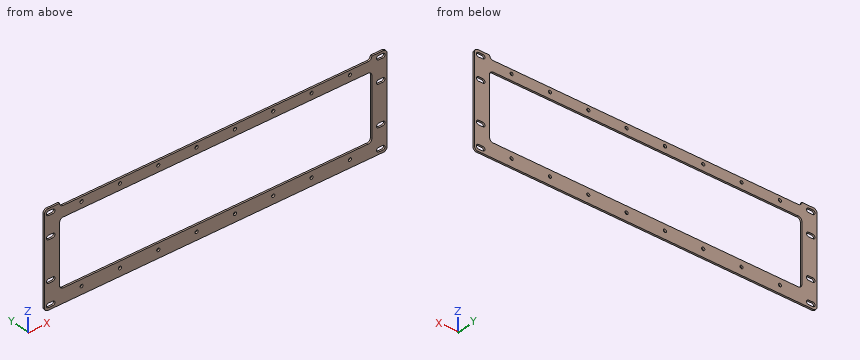
from build123d import *

# Parameters (mm, degrees)
F1_R     = 2.25
F2_DEPTH = 2.5


with BuildPart() as f2:
    # F1 (on face) → F2 (new body)
    with BuildSketch(Plane.XZ):
        with BuildLine():
            Line((241.3, -61.675), (241.3, 61.675))
            ThreePointArc((241.3, 61.675), (239.8355339059, 65.2105339059), (236.3, 66.675))
            Line((236.3, 66.675), (220, 66.675))
            ThreePointArc((220, 66.675), (218.5355339059, 63.1394660941), (215, 61.675))
            Line((215, 61.675), (-215, 61.675))
            ThreePointArc((-215, 61.675), (-218.5355339059, 63.1394660941), (-220, 66.675))
            Line((-220, 66.675), (-236.3, 66.675))
            ThreePointArc((-236.3, 66.675), (-239.8355339059, 65.2105339059), (-241.3, 61.675))
            Line((-241.3, 61.675), (-241.3, -61.675))
            ThreePointArc((-241.3, -61.675), (-239.8355339059, -65.2105339059), (-236.3, -66.675))
            Line((-236.3, -66.675), (236.3, -66.675))
            ThreePointArc((236.3, -66.675), (239.8355339059, -65.2105339059), (241.3, -61.675))
        make_face()
        with BuildLine():
            Line((-235.5, -57.4), (-229.5, -57.4))
            ThreePointArc((-229.5, -57.4), (-226.5, -60.4), (-229.5, -63.4))
            Line((-229.5, -63.4), (-235.5, -63.4))
            ThreePointArc((-235.5, -63.4), (-238.5, -60.4), (-235.5, -57.4))
        make_face(mode=Mode.SUBTRACT)
        with Locations((-189, -55.5)):
            Circle(F1_R, mode=Mode.SUBTRACT)
        with Locations((-135, -55.5)):
            Circle(F1_R, mode=Mode.SUBTRACT)
        with Locations((-81, -55.5)):
            Circle(F1_R, mode=Mode.SUBTRACT)
        with Locations((-27, -55.5)):
            Circle(F1_R, mode=Mode.SUBTRACT)
        with BuildLine():
            Line((-235.5, -25.6), (-229.5, -25.6))
            ThreePointArc((-229.5, -25.6), (-226.5, -28.6), (-229.5, -31.6))
            Line((-229.5, -31.6), (-235.5, -31.6))
            ThreePointArc((-235.5, -31.6), (-238.5, -28.6), (-235.5, -25.6))
        make_face(mode=Mode.SUBTRACT)
        with Locations((27, -55.5)):
            Circle(F1_R, mode=Mode.SUBTRACT)
        with Locations((81, -55.5)):
            Circle(F1_R, mode=Mode.SUBTRACT)
        with Locations((135, -55.5)):
            Circle(F1_R, mode=Mode.SUBTRACT)
        with BuildLine():
            Line((229.5, -57.4), (235.5, -57.4))
            ThreePointArc((235.5, -57.4), (238.5, -60.4), (235.5, -63.4))
            Line((235.5, -63.4), (229.5, -63.4))
            ThreePointArc((229.5, -63.4), (226.5, -60.4), (229.5, -57.4))
        make_face(mode=Mode.SUBTRACT)
        with Locations((189, -55.5)):
            Circle(F1_R, mode=Mode.SUBTRACT)
        with BuildLine():
            Line((229.5, -25.6), (235.5, -25.6))
            ThreePointArc((235.5, -25.6), (238.5, -28.6), (235.5, -31.6))
            Line((235.5, -31.6), (229.5, -31.6))
            ThreePointArc((229.5, -31.6), (226.5, -28.6), (229.5, -25.6))
        make_face(mode=Mode.SUBTRACT)
        with BuildLine():
            Line((-235.5, 31.6), (-229.5, 31.6))
            ThreePointArc((-229.5, 31.6), (-226.5, 28.6), (-229.5, 25.6))
            Line((-229.5, 25.6), (-235.5, 25.6))
            ThreePointArc((-235.5, 25.6), (-238.5, 28.6), (-235.5, 31.6))
        make_face(mode=Mode.SUBTRACT)
        with Locations((-189, 55.5)):
            Circle(F1_R, mode=Mode.SUBTRACT)
        with BuildLine():
            Line((-235.5, 63.4), (-229.5, 63.4))
            ThreePointArc((-229.5, 63.4), (-226.5, 60.4), (-229.5, 57.4))
            Line((-229.5, 57.4), (-235.5, 57.4))
            ThreePointArc((-235.5, 57.4), (-238.5, 60.4), (-235.5, 63.4))
        make_face(mode=Mode.SUBTRACT)
        with Locations((-135, 55.5)):
            Circle(F1_R, mode=Mode.SUBTRACT)
        with Locations((-81, 55.5)):
            Circle(F1_R, mode=Mode.SUBTRACT)
        with Locations((-27, 55.5)):
            Circle(F1_R, mode=Mode.SUBTRACT)
        with BuildLine():
            Line((-215, 46.5), (215, 46.5))
            ThreePointArc((215, 46.5), (218.5355339059, 45.0355339059), (220, 41.5))
            Line((220, 41.5), (220, -41.5))
            ThreePointArc((220, -41.5), (218.5355339059, -45.0355339059), (215, -46.5))
            Line((215, -46.5), (-215, -46.5))
            ThreePointArc((-215, -46.5), (-218.5355339059, -45.0355339059), (-220, -41.5))
            Line((-220, -41.5), (-220, 41.5))
            ThreePointArc((-220, 41.5), (-218.5355339059, 45.0355339059), (-215, 46.5))
        make_face(mode=Mode.SUBTRACT)
        with BuildLine():
            Line((229.5, 31.6), (235.5, 31.6))
            ThreePointArc((235.5, 31.6), (238.5, 28.6), (235.5, 25.6))
            Line((235.5, 25.6), (229.5, 25.6))
            ThreePointArc((229.5, 25.6), (226.5, 28.6), (229.5, 31.6))
        make_face(mode=Mode.SUBTRACT)
        with Locations((27, 55.5)):
            Circle(F1_R, mode=Mode.SUBTRACT)
        with Locations((81, 55.5)):
            Circle(F1_R, mode=Mode.SUBTRACT)
        with Locations((135, 55.5)):
            Circle(F1_R, mode=Mode.SUBTRACT)
        with Locations((189, 55.5)):
            Circle(F1_R, mode=Mode.SUBTRACT)
        with BuildLine():
            Line((229.5, 63.4), (235.5, 63.4))
            ThreePointArc((235.5, 63.4), (238.5, 60.4), (235.5, 57.4))
            Line((235.5, 57.4), (229.5, 57.4))
            ThreePointArc((229.5, 57.4), (226.5, 60.4), (229.5, 63.4))
        make_face(mode=Mode.SUBTRACT)
    extrude(amount=F2_DEPTH)


solid = f2.part
The listing builds one solid part. Answer for the finished solid, in the listing's coordinates (mm). Give positions to 0.01 mm unless a question says otherwise; leave off trailing zeros. Write each loop counter-clockwise with the first axis right and the second up, starting at its lowest first coordinate (ties: lowest second). Pieces come first, ordered by that corner, then holes. Notation, with made-up numbers: (77.25, 14.5) -> (107.25, 14.5) arc R11 cw to (107.25, 18.5) -> close; hole circle Ø6 at (55.25, -7.5). An arc over 180 degrees is marked (long way). One line per question, with ' | ' between items. Start each with the question number.
1. Section B-B (x = 171.5) is taken. Determine the outline of the cut face in (y, z) (3 decimals).
2. Section A-A (z = -18) is taken. Determine the outline of the cut face in (x, y), plus the area to 4 significant figures.
3. Section C-C (y = -1.95) is taken. State how many separate pieces and enclosed holes the cut face has, plus the area to 3 significant figures.
4. Find the intervals of material crossed by probe 1 along Z at (x, y) = (81, -1.15) (3 decimals); probe 2 along Z at (x, y) = (207.5, -2.2) (3 decimals); probe 3 along X at (y, z) = (-1.55, 61.5), in increasing order.
5. Given pin 1 Ø2.5 at (x, z) = (-189, 55.5) entering from -Y, flat-ended and moving along its own axis, determine where the tip first touches the part or whether it passes through.
Response values:
1) outline: (-2.5, -66.675) -> (0, -66.675) -> (0, -46.5) -> (-2.5, -46.5) -> close; (-2.5, 46.5) -> (0, 46.5) -> (0, 61.675) -> (-2.5, 61.675) -> close
2) outline: (-241.3, -2.5) -> (-220, -2.5) -> (-220, 0) -> (-241.3, 0) -> close; (220, -2.5) -> (241.3, -2.5) -> (241.3, 0) -> (220, 0) -> close | area: 106.5 mm2
3) separate pieces: 1 | enclosed holes: 25 | area: 20,500 mm2
4) probe 1: -66.675 to -57.75, -53.25 to -46.5, 46.5 to 53.25, 57.75 to 61.675 | probe 2: -66.675 to -46.5, 46.5 to 61.675 | probe 3: -241.3 to -238.29, -226.71 to 226.71, 238.29 to 241.3
5) pin 1: through
